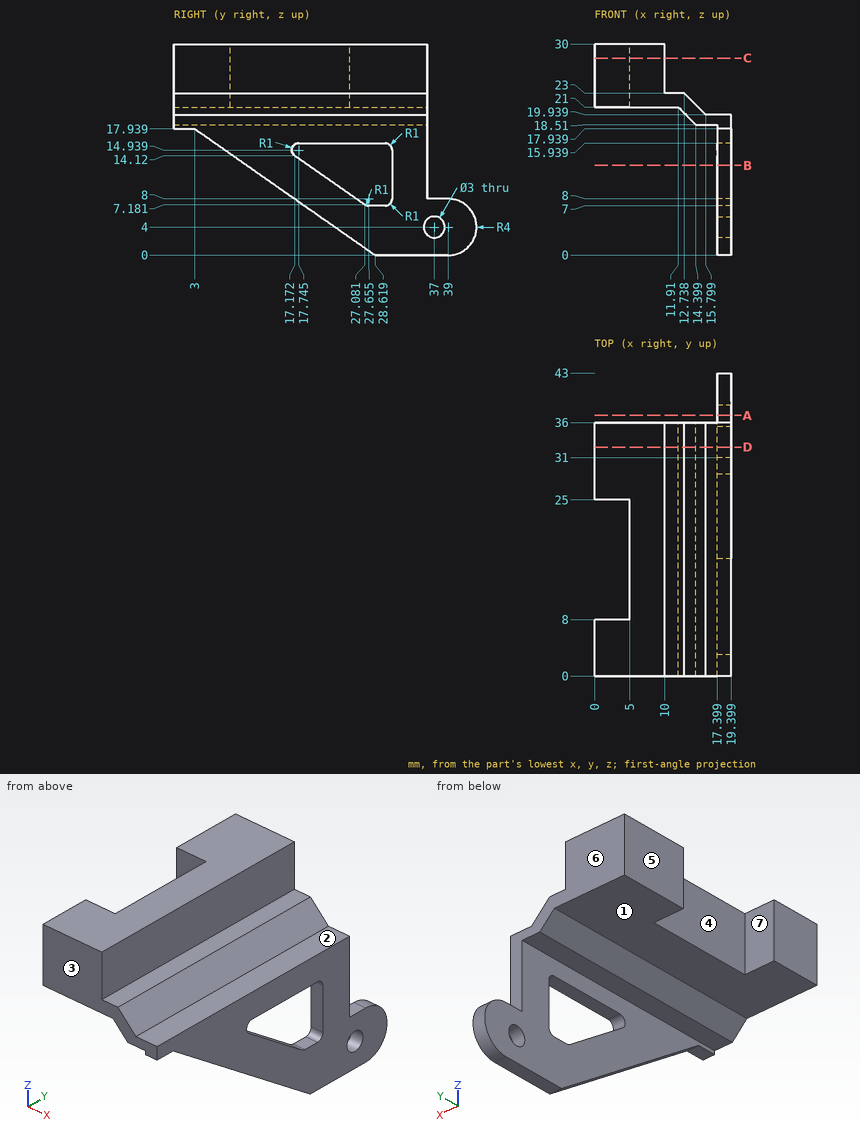
Could you check a few things on this drawing? It's one solid part, dimensions in mm from its lowest x, y, z. A direction names the side the tool comes from. Coordinates: 2 decimals unless noted, no trailing zeros. Order: outer loops, then holes, each group sorted by start corner. A loop starts at its lowest first (then second) coordinate and runs counter-clockwise, first axis right, second up. Notation, with made-up numbers: M -0.5,67 L 31.5,67 A24 cw 31.5,104 Z; hole C -24.5,87 d9. An arc over 180 degrees is marked long. Answer as a JSON object with one key per item and string values. Group by question number.
(1) I need wall thicknesses on probe 1 along Z at (x, y) = (1.75, 28.5); probe 2 along X at (y, z) = (31.5, 12.25); probe 3 along Z at (x, y) = (16.25, 14). Which ranges of each line are inside material? Lowest first, please.
(2) Which directions (+Z, -Z, +X, -X, +Y, -Y) give clear straight access to the entire face, cutting with the end or side of a thin tool? Please do the marked faces 1, 2, 3 and 4.
(3) Suppose I cut it at A-A, the plane y = 37. Please give me the cut outline in (x, z), then the cut area to 3 significant figures.
(4) Suppose I cut it at B-B, the plane z = 12.75. Please give me the cut outline in (x, y).
(5) For pin 1 (7 mm diameter, centred on y = 15.5, z = 23.5, fed in from -X); pin 2 (10 mm diameter, centred on x = 8, z = 13, fed in from +Y); pin 3 (0.6 mm diameter, centred on x = 19, z = 12.5, fed in from -Y); pin 4 (2 mm diameter, centred on y = 25.5, z = 26, fed in from +X), each with a flat end and sliding along its axis, tell me the tip position at first contact or that it passes through.
(6) Suppose I cut it at C-C, the plane z = 28. Please give me the cut outline in (x, y).
(7) If we mould it in two halves opening along Y, with no side actions, what happens to the marked faces 5, 6 and 7? For each: released by +Y, released by -Y, zero draft, split by the parting line, or undercut.
(8) Suppose I cut it at D-D, the plane y = 32.5. Please give me the cut outline in (x, z).
Values found:
{
 "1": {"probe 1": "z = 21 to 30", "probe 2": "x = 17.4 to 19.4", "probe 3": "z = 18.51 to 19.94"},
 "2": {"face 1": "-Z, -X, +Y, -Y", "face 2": "+Z, +X, +Y, -Y", "face 3": "+Z, -Z, +X, -X, -Y", "face 4": "+Z, -Z, -X"},
 "3": {"outline": "M 17.4,0 L 19.4,0 L 19.4,2.5 L 17.4,2.5 Z; M 17.4,5.5 L 19.4,5.5 L 19.4,8 L 17.4,8 Z", "area": "10.0 mm^2"},
 "4": {"outline": "M 17.4,10.41 L 19.4,10.41 L 19.4,19.13 L 17.4,19.13 Z; M 17.4,31 L 19.4,31 L 19.4,36 L 17.4,36 Z"},
 "5": {"pin 1": "stops at x = 5", "pin 2": "passes through", "pin 3": "stops at y = 10.34", "pin 4": "stops at x = 10"},
 "6": {"outline": "M 0,0 L 10,0 L 10,36 L 0,36 L 0,25 L 5,25 L 5,8 L 0,8 Z"},
 "7": {"face 5": "zero draft", "face 6": "released by +Y", "face 7": "undercut"},
 "8": {"outline": "M 0,21 L 11.91,21 L 14.4,18.51 L 17.4,18.51 L 17.4,0 L 19.4,0 L 19.4,19.94 L 15.8,19.94 L 12.74,23 L 10,23 L 10,30 L 0,30 Z"}
}
